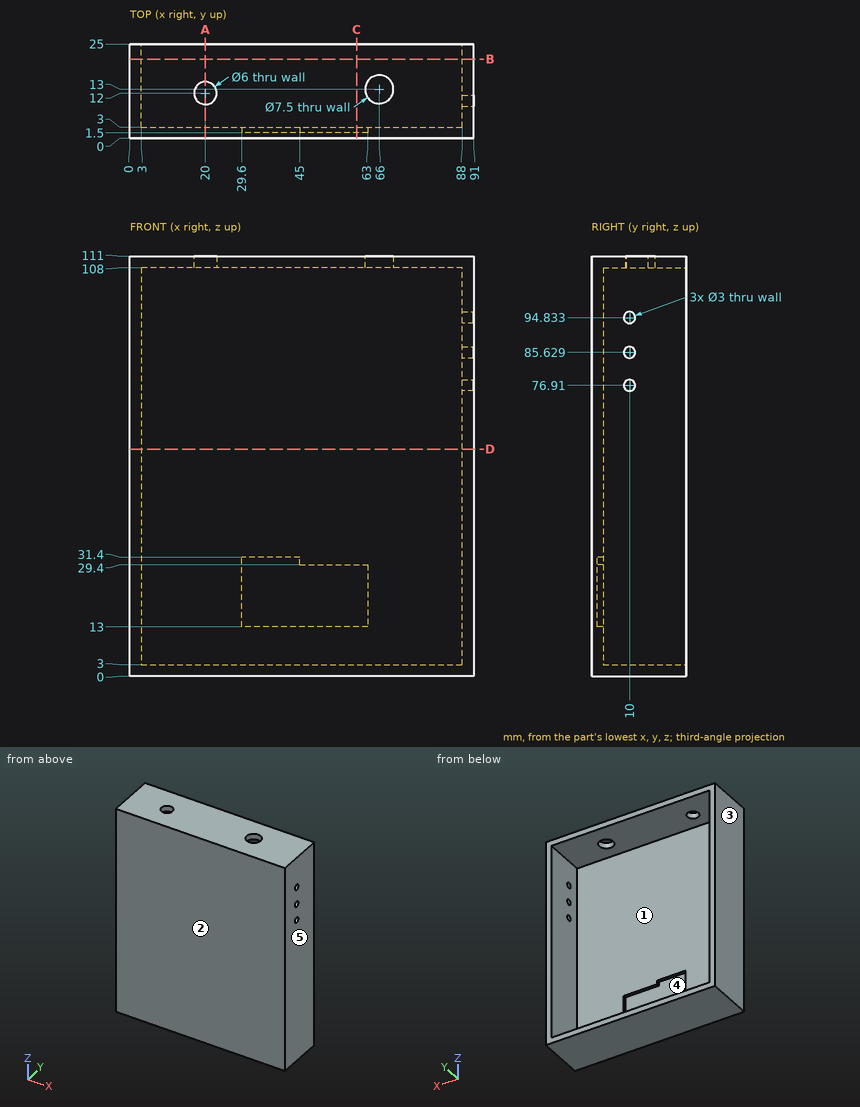
Source: three-view drawing plus pictorial views. Frame: mm from the lowest corner of the part. A direction names the side the tool comes from. Round coordinates to 2 decimals unless told otherwise and drop trailing zeros. Order: outer loops, then holes, each group sorted by start corner. A loop starts at its lowest first (then second) coordinate and runs counter-clockwise, first axis right, second up. Notation, with made-up numbers: (74.5, 81.5) - (114.5, 81.5) arc R17 ccw to (114.5, 107.5) - close; hole circle Ø2 at (75.5, 52). An arc over 180 degrees is marked (long way). Answer in a Markdown table with one row per item.
Item 1: Reachability of the marked faces 1 and 2 from +Z, -Z, +X, -X, +Y, -Y: full face, straight path, thin tool, end or side. Return the list, or none.
Model answer:
| item | result |
|---|---|
| face 1 | +Y |
| face 2 | +Z, -Z, +X, -X, -Y |
Item 2: Pin query (flat end, axial travel): pin 1 (1.8 mm diameter, centred on y = 10, z = 85.63, fed in from +X); pin 2 (5 mm diameter, centred on x = 15, z = 87.5, fed in from +Y); pin 3 (5.5 mm diameter, centred on x = 20, y = 12, fed in from +Z). Return the tip coordinate at first contact, or that it passes through.
Model answer:
| item | result |
|---|---|
| pin 1 | stops at x = 3 |
| pin 2 | stops at y = 3 |
| pin 3 | stops at z = 3 |
Item 3: Section query B-B (y = 21). Return the cut outline in (x, z), then the cut area to 3 significant figures.
Model answer:
| item | result |
|---|---|
| outline | (0, 0) - (91, 0) - (91, 111) - (0, 111) - close; hole (3, 3) - (88, 3) - (88, 108) - (3, 108) - close |
| area | 1,180 mm² |
Item 4: Section query D-D (z = 60). Return the cut outline in (x, y).
Model answer:
| item | result |
|---|---|
| outline | (0, 0) - (91, 0) - (91, 25) - (88, 25) - (88, 3) - (3, 3) - (3, 25) - (0, 25) - close |
Item 5: Section query C-C (x = 60). Return the cut outline in (y, z).
Model answer:
| item | result |
|---|---|
| outline | (0, 0) - (25, 0) - (25, 3) - (3, 3) - (3, 13) - (1.5, 13) - (1.5, 29.4) - (3, 29.4) - (3, 108) - (25, 108) - (25, 111) - (0, 111) - close |
Item 6: Line query: line 1 (Y direction, x = 66, z = 109); line 2 (X direction, y = 15, z = 72); line 3 (Z direction, x = 12, y = 14.75). Output: solid intervals per line, ascending.
Model answer:
| item | result |
|---|---|
| line 1 | y = 0 to 9.25, 16.75 to 25 |
| line 2 | x = 0 to 3, 88 to 91 |
| line 3 | z = 0 to 3, 108 to 111 |
Item 7: Mould query, pull axis X, two halves, no side actions, for the marked faces 3, 4 and 5. Classes: released by +X, released by -X, zero draft, split by the parting line, or undercut.
Model answer:
| item | result |
|---|---|
| face 3 | released by -X |
| face 4 | undercut |
| face 5 | released by +X |
Item 8: Section query A-A (x = 20). Return the cut outline in (y, z), then the cut area to 3 significant figures.
Model answer:
| item | result |
|---|---|
| outline | (0, 0) - (25, 0) - (25, 3) - (3, 3) - (3, 108) - (9, 108) - (9, 111) - (0, 111) - close; (15, 108) - (25, 108) - (25, 111) - (15, 111) - close |
| area | 447 mm² |
